Geometry: final body of the model. Coordinates: model frame, mm. Face numbers are marked on the shaded views. A direction names the side the tool comes from. Round coordinates to 2 decimals unless told otherwise and drop trailing zeros. Order: outer loops, then holes, each group sorted by start corner. A loop starts at its lowest first (then second) coordinate and runs counter-clockwise, first axis right, second up. Notation, with made-up numbers: M 78.25,0.5 L 98.25,0.5 A32 ccw 98.25,34.5 Z; hole C 68.25,15 d3. An arc over 180 degrees is marked long. Return JSON: item names as keys, results as strings. Group by question number.
Q1. Mould query, pull axis Y, two halves, no side actions, for the marked faces 1, 2, 3 and 4. Classes: released by +Y, released by -Y, zero draft, split by the parting line, or undercut.
Q2. Ray query, probe 1 along Y at (x, z) = (0, 0.6); probe 2 along Z at (x, y) = (3.5, -49); probe 3 along Z at (x, y) = (5, -51). Return the intervals inside material, ascending.
Q3. Cut plane A-A on x = 0. Output: boundary loops of the cut face in (y, z).
Q4. Cut plane B-B on y = -49.25. Output: boundary loops of the cut face in (x, z).
Q5. Cut plane D-D on z = 25. Output: boundary loops of the cut face in (x, y), and give its area (3 significant figures).
Q6. Access query for the marked faces 5, 6, 7 and 8. Directions: +Z, -Z, +X, -X, +Y, -Y. A direction counts if a zero-diameter tool reaches every point of the face in a straight line with its end or side. Return the directions, or none.
Q7. Cut plane C-C on y = -34. Output: boundary loops of the cut face in (x, z).
Q8. Contact query for flat-ended pins moving along their axis: pin 1 (1.5 mm diameter, centred on x = 0.5, z = 22.5, fed in from +Y); pin 2 (8.5 mm diameter, centred on y = -45, z = 23, fed in from -X); pin 3 (3 mm diameter, centred on x = 4, z = 11.5, fed in from +Y); pin 4 (4 mm diameter, centred on x = 0, y = -43.01, fed in from +Z). Output: stop coordinate, or through.
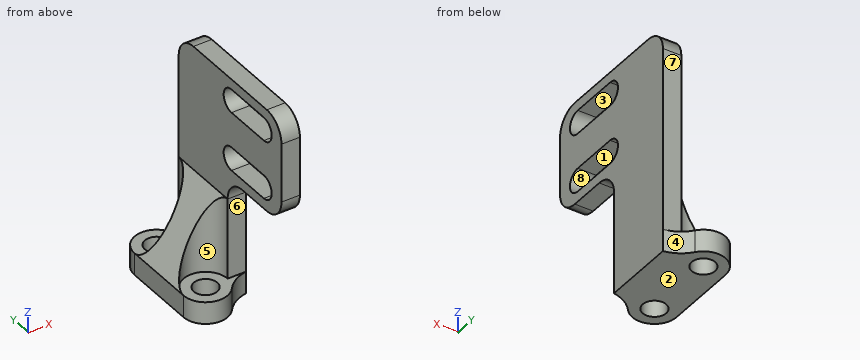
```python
from build123d import *

# Parameters (mm, degrees)
SKETCH_1_R          = 1.6
EXTRUDE_1_DEPTH     = 3
SKETCH_3_W          = 2.5
SKETCH_3_H          = 10
EXTRUDE_2_DEPTH     = 28
FILLET_1_R          = 5
FILLET_2_R          = 5
SKETCH_4_W          = 14
SKETCH_4_H          = 11
EXTRUDE_3_DEPTH     = 2.5
CUT_EXTRUDE_1_DEPTH = 63.851944341
EXTRUDE_4_DEPTH     = 10
SKETCH_8_R          = 3
CUT_EXTRUDE_2_DEPTH = 62.084915548
FILLET_3_R          = 3


with BuildPart() as part:
    # 草图1 → 凸台-拉伸1 (new body)
    with BuildSketch(Plane.XY):
        with BuildLine():
            ThreePointArc((3, -33.010340746), (0, -30.010340746), (-3, -33.010340746))
            Line((-3, -33.010340746), (-3, -43.010340746))
            ThreePointArc((-3, -43.010340746), (0, -46.010340746), (3, -43.010340746))
            Line((3, -43.010340746), (5.5, -43.010340746))
            Line((5.5, -43.010340746), (5.5, -33.010340746))
            Line((5.5, -33.010340746), (3, -33.010340746))
        make_face()
        with Locations((0, -33.010340746)):
            Circle(SKETCH_1_R, mode=Mode.SUBTRACT)
        with Locations((0, -43.010340746)):
            Circle(SKETCH_1_R, mode=Mode.SUBTRACT)
    extrude(amount=EXTRUDE_1_DEPTH)

    # 草图3 → 凸台-拉伸2 (add)
    with BuildSketch(Plane.XY.offset(3)):
        with Locations((4.25, -38.010340746)):
            Rectangle(SKETCH_3_W, SKETCH_3_H)
    extrude(amount=EXTRUDE_2_DEPTH)

    # 圆角1
    # the kernel refuses this fillet: 5 mm, written as the material it adds along each edge
    with BuildSketch(Plane(origin=(3, -43.010340746, 0), x_dir=(-0.32639560491693326, -0.9452332564456825, 0), z_dir=(0, 0, 1))) as fillet_1_piece_1:
        with BuildLine():
            CenterArc((3.590351654, 4.726166282), FILLET_1_R, 208.20428203, 42.745569225)
            Line((-0.815989012, 2.363083141), (0, 0))
            ThreePointArc((0, 0), (0.979186815, 0.164300231), (1.95837363, 0))
        make_face()
    extrude(amount=3)

    # 圆角2
    # the kernel refuses this fillet: 5 mm, written as the material it adds along each edge
    with BuildSketch(Plane(origin=(3, -33.010340746, 0), x_dir=(1, 0, 0), z_dir=(0, 0, 1))) as fillet_2_piece_1:
        with BuildLine():
            CenterArc((3.295454545, 4.936319688), FILLET_2_R, 218.100297491, 42.745569225)
            ThreePointArc((-0.639204545, 1.851119883), (-0.164300231, 0.979186815), (0, 0))
            Line((0, 0), (2.5, 0))
        make_face()
    extrude(amount=3)

    # 草图4 → 凸台-拉伸3 (add)
    with BuildSketch(Plane(origin=(5.5, 0, 0), x_dir=(0, 0, -1), z_dir=(1, 0, 0))):
        with Locations((-24, -48.510340746)):
            Rectangle(SKETCH_4_W, SKETCH_4_H)
    extrude(amount=-EXTRUDE_3_DEPTH)

    # 草图5 → 切除-拉伸1 (cut, through all)
    with BuildSketch(Plane(origin=(5.5, 0, 0), x_dir=(0, 0, -1), z_dir=(1, 0, 0))):
        with BuildLine():
            Line((-26.4, -50.402762968), (-26.4, -43.797439087))
            ThreePointArc((-26.4, -43.797439087), (-28, -42.197439087), (-29.6, -43.797439087))
            Line((-29.6, -43.797439087), (-29.6, -50.402762968))
            ThreePointArc((-29.6, -50.402762968), (-28, -52.002762968), (-26.4, -50.402762968))
        make_face()
        with BuildLine():
            Line((-21.6, -50.402762968), (-21.6, -43.797439087))
            ThreePointArc((-21.6, -43.797439087), (-20, -42.197439087), (-18.4, -43.797439087))
            Line((-18.4, -43.797439087), (-18.4, -50.402762968))
            ThreePointArc((-18.4, -50.402762968), (-20, -52.002762968), (-21.6, -50.402762968))
        make_face()
    extrude(amount=-CUT_EXTRUDE_1_DEPTH, mode=Mode.SUBTRACT)

    # 草图6 → 凸台-拉伸4 (add)
    with BuildSketch(Plane.XZ.offset(43.010340746)):
        Polygon((3, 14), (-3, 3), (3, 3), align=None)
    extrude(amount=-EXTRUDE_4_DEPTH)

    # 草图8 → 切除-拉伸2 (cut, through all)
    with BuildSketch(Plane.XY.offset(3)):
        with Locations((0, -43.010340746)):
            Circle(SKETCH_8_R)
        with Locations((0, -33.010340746)):
            Circle(SKETCH_8_R)
    extrude(amount=CUT_EXTRUDE_2_DEPTH, mode=Mode.SUBTRACT)

    # 圆角3
    fillet_3_edges = [part.edges().sort_by_distance(p)[0] for p in [
        (4.25, -43.010340746, 17),
        (4.25, -54.010340746, 17),
        (4.25, -54.010340746, 31),
        (4.25, -33.010340746, 31),
    ]]
    fillet(fillet_3_edges, radius=FILLET_3_R)


solid = part.part
```
Result sheet:
{
 "1": {"face 1": "undercut", "face 2": "zero draft", "face 3": "undercut", "face 4": "released by +Y"},
 "2": {"probe 1": "y = -46.01 to -44.61, -41.41 to -34.61, -31.41 to -30.01", "probe 2": "z = 17 to 18.4, 21.6 to 26.4, 29.6 to 31", "probe 3": "z = 17 to 18.52, 21.48 to 26.52, 29.48 to 31"},
 "3": {"outline": "M -46.01,0 L -44.61,0 L -44.61,3 L -46.01,3 Z; M -41.41,0 L -34.61,0 L -34.61,3 L -36.01,3 L -36.01,8.5 L -40.01,8.5 L -40.01,3 L -41.41,3 Z; M -31.41,0 L -30.01,0 L -30.01,3 L -31.41,3 Z"},
 "4": {"outline": "M 3,17 L 5.5,17 L 5.5,18.4 L 3,18.4 Z; M 3,21.6 L 5.5,21.6 L 5.5,26.4 L 3,26.4 Z; M 3,29.6 L 5.5,29.6 L 5.5,31 L 3,31 Z"},
 "5": {"outline": "M 3,-54.01 L 5.5,-54.01 L 5.5,-33.01 L 3,-33.01 Z", "area": "52.5 mm²"},
 "6": {"face 5": "+Z, -Y", "face 6": "+X, -X, -Y", "face 7": "+Z, +X, -X, +Y", "face 8": "+X, -X"},
 "7": {"outline": "M -3,0 L -1.26,0 L -1.26,3 L -2.83,3 L -2.83,3.31 L -3,3 Z; M 1.26,0 L 5.5,0 L 5.5,30.23 L 3,30.23 L 3,14 L 2.83,13.69 L 2.83,3 L 1.26,3 Z"},
 "8": {"pin 1": "passes through", "pin 2": "stops at x = 3", "pin 3": "stops at y = -33.01", "pin 4": "stops at z = 3"}
}
